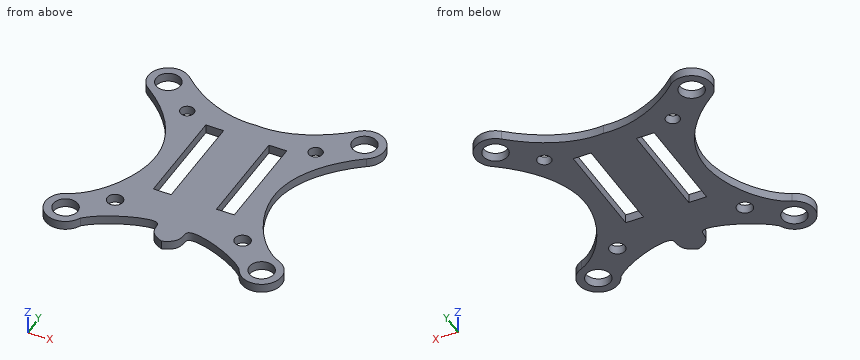
```python
from build123d import *

# Parameters (mm, degrees)
F0_R     = 0.6985
F0_R_2   = 0.4455322906
F0_W     = 1.0151027236
F0_H     = 5.8303333353
F0_R_3   = 0.3904241603
F1_DEPTH = 0.508


with BuildPart() as f1:
    # F0 (on Top) → F1 (new body)
    with BuildSketch(Plane.XY):
        with BuildLine():
            add(Edge.make_bspline(
                [(-4.8071383511, 6.5496880167), (-3.5494174307, 5.3943343251), (-1.775382203, 4.4622034766), (0, 4.6114819124)],
                knots=[0, 0, 0, 0, 5.1831671813, 5.1831671813, 5.1831671813, 5.1831671813], degree=3))
            ThreePointArc((-4.8071383511, 6.5496880167), (-6.4941252197, 6.4116965525), (-6.1940324141, 4.7458902471))
            add(Edge.make_bspline(
                [(-6.1940324141, 4.7458902471), (-4.693901011, 3.6446792104), (-2.0902496032, 0.2759509244), (-4.6702187254, -4.0639645625), (-5.9934721436, -4.646336657)],
                knots=[0, 0, 0, 0, 0.5042985744, 1, 1, 1, 1], degree=3))
            ThreePointArc((-5.9934721436, -4.646336657), (-6.4052483977, -6.5140957742), (-4.5287124963, -6.1443704514))
            add(Edge.make_bspline(
                [(-4.5287124963, -6.1443704514), (-3.6492146823, -5.2652203685), (0.1529797259, -3.8611909007), (-1.1026566893, -5.5442661801), (0, -5.9233158827)],
                knots=[0, 0, 0, 0, 0.6177222982, 1, 1, 1, 1], degree=3))
            add(Edge.make_bspline(
                [(4.5287124963, -6.1443704514), (3.6492146823, -5.2652203685), (-0.1529797259, -3.8611909007), (1.1026566893, -5.5442661801), (0, -5.9233158827)],
                knots=[0, 0, 0, 0, 0.6177222982, 1, 1, 1, 1], degree=3))
            ThreePointArc((4.5287124963, -6.1443704514), (6.4052483977, -6.5140957742), (5.9934721436, -4.646336657))
            add(Edge.make_bspline(
                [(6.1940324141, 4.7458902471), (4.693901011, 3.6446792104), (2.0902496032, 0.2759509244), (4.6702187254, -4.0639645625), (5.9934721436, -4.646336657)],
                knots=[0, 0, 0, 0, 0.5042985744, 1, 1, 1, 1], degree=3))
            ThreePointArc((6.1940324141, 4.7458902471), (6.4941252197, 6.4116965525), (4.8071383511, 6.5496880167))
            add(Edge.make_bspline(
                [(4.8071383511, 6.5496880167), (3.5494174307, 5.3943343251), (1.775382203, 4.4622034766), (0, 4.6114819124)],
                knots=[0, 0, 0, 0, 5.1831671813, 5.1831671813, 5.1831671813, 5.1831671813], degree=3))
        make_face()
        with Locations((-5.588, -5.715)):
            Circle(F0_R, mode=Mode.SUBTRACT)
        with Locations((-3.6327592097, -4.0190205909)):
            Circle(F0_R_2, mode=Mode.SUBTRACT)
        with Locations((5.588, -5.715)):
            Circle(F0_R, mode=Mode.SUBTRACT)
        with Locations((3.6327592097, -4.0190205909)):
            Circle(F0_R_2, mode=Mode.SUBTRACT)
        with Locations((-1.7977658426, 0.5619557342)):
            Rectangle(F0_W, F0_H, mode=Mode.SUBTRACT)
        with Locations((-3.6587875802, 4.049744457)):
            Circle(F0_R_3, mode=Mode.SUBTRACT)
        with Locations((-5.588, 5.715)):
            Circle(F0_R, mode=Mode.SUBTRACT)
        with Locations((1.7977658426, 0.5619557342)):
            Rectangle(F0_W, F0_H, mode=Mode.SUBTRACT)
        with Locations((3.6587875802, 4.049744457)):
            Circle(F0_R_3, mode=Mode.SUBTRACT)
        with Locations((5.588, 5.715)):
            Circle(F0_R, mode=Mode.SUBTRACT)
    extrude(amount=F1_DEPTH)


solid = f1.part
```
Here's how the part is built. I have some questions about the finished solid (model axes, mm). Give positions to 0.01 mm unless a question says otherwise; leave off trailing zeros. Put each result on its own line as item: value. Start each with the question number.
(1) I need wall thicknesses on line 1 along X through (y, z) = (4, 0.35); line 2 along X through (y, z) = (0.5, 0.1); line 3 along Y through (x, z) = (6, 0.2). Which ranges of each line are inside material? Lowest first, please. Write a range as [from, to].
(2) I want a section at A-A on x = -3.75. State how many separate pieces and enclosed holes the cut face has, then the cut area to 3 significant figures.
(3) Will this pin go through, and if not, where does the flat tip stop? pin 1 Ø0.8 at (x, y) = (-5.588, -5.715) entering from -Z.
Answer block:
1. line 1: [-5.31, -4.05], [-3.27, 3.27], [4.05, 5.31]
1. line 2: [-3.41, -2.31], [-1.29, 1.29], [2.31, 3.41]
1. line 3: [-6.78, -6.28], [-5.15, -4.65], [4.6, 5.15], [6.28, 6.78]
2. separate pieces: 4
2. enclosed holes: 0
2. area: 3.06 mm^2
3. pin 1: through
